Geometry: final body of the model. Coordinates: model frame, mm. Coordinates: 2 decimals unless noted, no trailing zeros. Order: outer loops, then holes, each group sorted by start corner. A loop starts at its lowest first (then second) coordinate and runs counter-clockwise, first axis right, second up. Notation, with made-up numbers: M -39.75,37 L -29.75,37 A18 cw -29.75,47 Z; hole C 87,-21.5 d1. An arc over 180 degrees is marked long. Use CSV: the item, a comma, the result in double quotes. Start each with the question number.
Q1. First-contact query: P1, Ø3.5, axis at x = -56.25, z = 83.5, coming from the +Y side; P2, Ø0.6, axis at y = -1, z = 104.5, coming from the +X side. Flat tips, straight axial feed; report the tip coordinate or a pass-through.
Q2. Section query B-B, the plane z = 6. Output: boundary loops of the cut face in (x, y).
Q3. Ray query, probe 1 along X at (y, z) = (-0.6, -33); probe 2 along X at (y, z) = (-0.95, 32); probe 3 along Z at (x, y) = (-7.25, -0.85). Return the intervals inside material, ascending.
Q4. Mould query, pull axis Z, two halves, no side actions, for faces 1 (the face through (-55.42, -0.99, 0.25)), 2 (the face through (-1, -2, 35)). Classes: +Z half, -Z half, draft (parallel to the pull), parting line (faces both ways), or undercut.
Q5. Section query A-A, the plane y = -0.3. State how many separate pieces and enclosed holes the cut face has, and give its area (3 significant figures).
from build123d import *

# Parameters (mm, degrees)
F0_R     = 1.5
F1_DEPTH = 2


with BuildPart() as f1:
    # F0 (on Front) → F1 (new body)
    with BuildSketch(Plane.XZ):
        with BuildLine():
            ThreePointArc((-46.5, 108.5), (-48.62132, 107.62132), (-49.5, 105.5))
            Line((-49.5, 105.5), (-49.5, 101.5))
            ThreePointArc((-49.5, 101.5), (-50.37868, 99.37868), (-52.5, 98.5))
            Line((-52.5, 98.5), (-65.5, 98.5))
            ThreePointArc((-65.5, 98.5), (-67.62132, 97.62132), (-68.5, 95.5))
            Line((-68.5, 95.5), (-68.5, 15.731583))
            ThreePointArc((-68.5, 15.731583), (-67.806689, 13.813462), (-66.047208, 12.781911))
            ThreePointArc((-66.047208, 12.781911), (-55.418443, 0), (-66.047208, -12.781911))
            ThreePointArc((-66.047208, -12.781911), (-67.806689, -13.813462), (-68.5, -15.731583))
            Line((-68.5, -15.731583), (-68.5, -37.032465))
            ThreePointArc((-68.5, -37.032465), (-67.62132, -39.153786), (-65.5, -40.032465))
            Line((-65.5, -40.032465), (65.5, -40.032465))
            ThreePointArc((65.5, -40.032465), (67.62132, -39.153786), (68.5, -37.032465))
            Line((68.5, -37.032465), (68.5, -16.733201))
            ThreePointArc((68.5, -16.733201), (67.800895, -14.808134), (66.029412, -13.780283))
            ThreePointArc((66.029412, -13.780283), (55.323529, -0.984306), (66.029412, 11.811671))
            ThreePointArc((66.029412, 11.811671), (67.800895, 12.839522), (68.5, 14.764589))
            Line((68.5, 14.764589), (68.5, 95.5))
            ThreePointArc((68.5, 95.5), (67.62132, 97.62132), (65.5, 98.5))
            Line((65.5, 98.5), (52.5, 98.5))
            ThreePointArc((52.5, 98.5), (50.37868, 99.37868), (49.5, 101.5))
            Line((49.5, 101.5), (49.5, 105.5))
            ThreePointArc((49.5, 105.5), (48.62132, 107.62132), (46.5, 108.5))
            Line((46.5, 108.5), (0, 108.5))
            Line((0, 108.5), (-46.5, 108.5))
        make_face()
        with BuildLine():
            ThreePointArc((-65.227546, -31.279437), (-65.25, -31), (-65.227546, -30.720563))
            Line((-65.227546, -30.720563), (-65.227546, -29.249952))
            ThreePointArc((-65.227546, -29.249952), (-63.477546, -27.499952), (-61.727546, -29.249952))
            Line((-61.727546, -29.249952), (-61.727546, -32.749317))
            ThreePointArc((-61.727546, -32.749317), (-63.477546, -34.499317), (-65.227546, -32.749317))
            Line((-65.227546, -32.749317), (-65.227546, -31.279437))
        make_face(mode=Mode.SUBTRACT)
        with BuildLine():
            ThreePointArc((-61.793502, 30.38777), (-61.76091, 30.195101), (-61.75, 30))
            ThreePointArc((-61.75, 30), (-61.76091, 29.804899), (-61.793502, 29.61223))
            Line((-61.793502, 29.61223), (-61.793502, 28.240838))
            ThreePointArc((-61.793502, 28.240838), (-63.543502, 26.490838), (-65.293502, 28.240838))
            Line((-65.293502, 28.240838), (-65.293502, 31.740202))
            ThreePointArc((-65.293502, 31.740202), (-63.543502, 33.490202), (-61.793502, 31.740202))
            Line((-61.793502, 31.740202), (-61.793502, 30.38777))
        make_face(mode=Mode.SUBTRACT)
        with Locations((-56.25, 25.5)):
            Circle(F0_R, mode=Mode.SUBTRACT)
        with Locations((-7.25, 25.5)):
            Circle(F0_R, mode=Mode.SUBTRACT)
        with Locations((1.25, -3.244149)):
            Circle(F0_R, mode=Mode.SUBTRACT)
        with BuildLine():
            ThreePointArc((65.227546, -30.720563), (65.244377, -30.859831), (65.25, -31))
            ThreePointArc((65.25, -31), (65.244377, -31.140169), (65.227546, -31.279437))
            Line((65.227546, -31.279437), (65.227546, -32.749317))
            ThreePointArc((65.227546, -32.749317), (63.477546, -34.499317), (61.727546, -32.749317))
            Line((61.727546, -32.749317), (61.727546, -29.249952))
            ThreePointArc((61.727546, -29.249952), (63.477546, -27.499952), (65.227546, -29.249952))
            Line((65.227546, -29.249952), (65.227546, -30.720563))
        make_face(mode=Mode.SUBTRACT)
        with Locations((49.5, -3.244149)):
            Circle(F0_R, mode=Mode.SUBTRACT)
        with BuildLine():
            ThreePointArc((61.793502, 29.61223), (61.75, 30), (61.793502, 30.38777))
            Line((61.793502, 30.38777), (61.793502, 31.740202))
            ThreePointArc((61.793502, 31.740202), (63.543502, 33.490202), (65.293502, 31.740202))
            Line((65.293502, 31.740202), (65.293502, 28.240838))
            ThreePointArc((65.293502, 28.240838), (63.543502, 26.490838), (61.793502, 28.240838))
            Line((61.793502, 28.240838), (61.793502, 29.61223))
        make_face(mode=Mode.SUBTRACT)
        with BuildLine():
            ThreePointArc((-65.230854, 53.741844), (-65.25, 54), (-65.230854, 54.258156))
            Line((-65.230854, 54.258156), (-65.230854, 55.701408))
            ThreePointArc((-65.230854, 55.701408), (-63.480854, 57.451408), (-61.730854, 55.701408))
            Line((-61.730854, 55.701408), (-61.730854, 52.202043))
            ThreePointArc((-61.730854, 52.202043), (-63.480854, 50.452043), (-65.230854, 52.202043))
            Line((-65.230854, 52.202043), (-65.230854, 53.741844))
        make_face(mode=Mode.SUBTRACT)
        with BuildLine():
            Line((-61.783352, 79.749682), (-61.783352, 78.340028))
            ThreePointArc((-61.783352, 78.340028), (-61.758358, 78.17083), (-61.75, 78))
            ThreePointArc((-61.75, 78), (-61.758358, 77.82917), (-61.783352, 77.659972))
            Line((-61.783352, 77.659972), (-61.783352, 76.250318))
            ThreePointArc((-61.783352, 76.250318), (-63.533352, 74.500318), (-65.283352, 76.250318))
            Line((-65.283352, 76.250318), (-65.283352, 79.749682))
            ThreePointArc((-65.283352, 79.749682), (-63.533352, 81.499682), (-61.783352, 79.749682))
        make_face(mode=Mode.SUBTRACT)
        with Locations((-56.25, 83.5)):
            Circle(F0_R, mode=Mode.SUBTRACT)
        with Locations((-7.25, 83.5)):
            Circle(F0_R, mode=Mode.SUBTRACT)
        with BuildLine():
            Line((-35.75, 104.75), (-34, 104.75))
            Line((-34, 104.75), (-32.25, 104.75))
            ThreePointArc((-32.25, 104.75), (-30.5, 103), (-32.25, 101.25))
            Line((-32.25, 101.25), (-34, 101.25))
            Line((-34, 101.25), (-35.75, 101.25))
            ThreePointArc((-35.75, 101.25), (-37.5, 103), (-35.75, 104.75))
        make_face(mode=Mode.SUBTRACT)
        with BuildLine():
            ThreePointArc((65.230854, 54.258156), (65.245207, 54.129432), (65.25, 54))
            ThreePointArc((65.25, 54), (65.245207, 53.870568), (65.230854, 53.741844))
            Line((65.230854, 53.741844), (65.230854, 52.202043))
            ThreePointArc((65.230854, 52.202043), (63.480854, 50.452043), (61.730854, 52.202043))
            Line((61.730854, 52.202043), (61.730854, 55.701408))
            ThreePointArc((61.730854, 55.701408), (63.480854, 57.451408), (65.230854, 55.701408))
            Line((65.230854, 55.701408), (65.230854, 54.258156))
        make_face(mode=Mode.SUBTRACT)
        with Locations((1.25, 71.655851)):
            Circle(F0_R, mode=Mode.SUBTRACT)
        with BuildLine():
            ThreePointArc((0.281149, 101.272732), (0, 101.25), (-0.281149, 101.272732))
            Line((-0.281149, 101.272732), (-1.743335, 101.272732))
            ThreePointArc((-1.743335, 101.272732), (-3.493335, 103.022732), (-1.743335, 104.772732))
            Line((-1.743335, 104.772732), (1.756665, 104.772732))
            ThreePointArc((1.756665, 104.772732), (3.506665, 103.022732), (1.756665, 101.272732))
            Line((1.756665, 101.272732), (0.281149, 101.272732))
        make_face(mode=Mode.SUBTRACT)
        with BuildLine():
            ThreePointArc((34.072565, 101.251505), (34, 101.25), (33.927435, 101.251505))
            Line((33.927435, 101.251505), (32.328993, 101.251505))
            ThreePointArc((32.328993, 101.251505), (30.578993, 103.001505), (32.328993, 104.751505))
            Line((32.328993, 104.751505), (35.828993, 104.751505))
            ThreePointArc((35.828993, 104.751505), (37.578993, 103.001505), (35.828993, 101.251505))
            Line((35.828993, 101.251505), (34.072565, 101.251505))
        make_face(mode=Mode.SUBTRACT)
        with Locations((49.5, 79.255851)):
            Circle(F0_R, mode=Mode.SUBTRACT)
        with BuildLine():
            ThreePointArc((61.783352, 77.659972), (61.75, 78), (61.783352, 78.340028))
            Line((61.783352, 78.340028), (61.783352, 79.749682))
            ThreePointArc((61.783352, 79.749682), (63.533352, 81.499682), (65.283352, 79.749682))
            Line((65.283352, 79.749682), (65.283352, 76.250318))
            ThreePointArc((65.283352, 76.250318), (63.533352, 74.500318), (61.783352, 76.250318))
            Line((61.783352, 76.250318), (61.783352, 77.659972))
        make_face(mode=Mode.SUBTRACT)
    extrude(amount=F1_DEPTH)


solid = f1.part
Responses:
1,P1,"stops at y = 0"
1,P2,"stops at x = 49.5"
2,outline,"M -56.89,-2 L 57.36,-2 L 57.36,0 L -56.89,0 Z"
3,probe 1,"x = -68.5 to -65.21, -61.75 to 61.75, 65.21 to 68.5"
3,probe 2,"x = -68.5 to -65.27, -61.81 to 61.81, 65.27 to 68.5"
3,probe 3,"z = -40.03 to 24, 27 to 82, 85 to 108.5"
4,face 1,"undercut"
4,face 2,"draft"
5,separate pieces,"1"
5,enclosed holes,"19"
5,area,"19,100 mm²"
